from build123d import *

# Parameters (mm, degrees)
SKETCH_1_R          = 1.7
SKETCH_1_W          = 5
SKETCH_1_H          = 13
SKETCH_1_H_2        = 2
EXTRUDE_3_DEPTH     = 2.9
SKETCH_3_R          = 2.1
CUT_EXTRUDE_3_DEPTH = 2.9


with BuildPart() as part:
    # 草图1 → 凸台-拉伸3 (new body)
    # profile 1 of 10: a face of its own
    with BuildSketch(Plane(origin=(0, 0, 0), x_dir=(1, 0, 0), z_dir=(0, 1, 0))):
        with BuildLine():
            Line((-40, 113), (-70, 113))
            Line((-70, 113), (-70, 108))
            Line((-70, 108), (-70, 92))
            Line((-70, 92), (-63.7, 92))
            ThreePointArc((-63.7, 92), (-62, 93.7), (-60.3, 92))
            ThreePointArc((-60.3, 92), (-60.797918472, 90.797918472), (-62, 90.3))
            Line((-62, 90.3), (-62, 87))
            Line((-62, 87), (-48, 87))
            Line((-48, 87), (-48, 90.3))
            ThreePointArc((-48, 90.3), (-49.202081528, 93.202081528), (-46.3, 92))
            Line((-46.3, 92), (-40, 92))
            Line((-40, 92), (-40, 113))
        make_face()
        with Locations(Location((-62, 108, 0), (0, 0, 270))):
            Circle(SKETCH_1_R, mode=Mode.SUBTRACT)
        with Locations(Location((-48, 108, 0), (0, 0, 270))):
            Circle(SKETCH_1_R, mode=Mode.SUBTRACT)
    # profile 2 of 10: a face of its own
    with BuildSketch(Plane(origin=(0, 0, 0), x_dir=(1, 0, 0), z_dir=(0, 1, 0))):
        with BuildLine():
            Line((-70, 92), (-70, 87))
            Line((-70, 87), (-62, 87))
            Line((-62, 87), (-62, 90.3))
            ThreePointArc((-62, 90.3), (-63.202081528, 90.797918472), (-63.7, 92))
            Line((-63.7, 92), (-70, 92))
        make_face()
    # profile 3 of 10: a face of its own
    with BuildSketch(Plane(origin=(0, 0, 0), x_dir=(1, 0, 0), z_dir=(0, 1, 0))):
        with BuildLine():
            Line((-48, 90.3), (-48, 87))
            Line((-48, 87), (-40, 87))
            Line((-40, 87), (-40, 92))
            Line((-40, 92), (-46.3, 92))
            ThreePointArc((-46.3, 92), (-46.797918472, 90.797918472), (-48, 90.3))
        make_face()
    # profile 4 of 10: a face of its own
    with BuildSketch(Plane(origin=(0, 0, 0), x_dir=(1, 0, 0), z_dir=(0, 1, 0))):
        Polygon((-70, 87), (-70, 80), (-20, 80), (-20, 85), (-25, 85), (-25, 87), (-40, 87), (-48, 87), (-62, 87), align=None)
    # profile 5 of 10: a face of its own
    with BuildSketch(Plane(origin=(0, 0, 0), x_dir=(1, 0, 0), z_dir=(0, 1, 0))):
        Polygon((-25, 113), (-40, 113), (-40, 92), (-40, 87), (-25, 87), (-25, 100), align=None)
    # profile 6 of 10: a face of its own
    with BuildSketch(Plane(origin=(0, 0, 0), x_dir=(1, 0, 0), z_dir=(0, 1, 0))):
        with Locations((-22.5, 93.5)):
            Rectangle(SKETCH_1_W, SKETCH_1_H)
    # profile 7 of 10: a face of its own
    with BuildSketch(Plane(origin=(0, 0, 0), x_dir=(1, 0, 0), z_dir=(0, 1, 0))):
        with Locations((-22.5, 106.5)):
            Rectangle(SKETCH_1_W, SKETCH_1_H)
    # profile 8 of 10: a face of its own
    with BuildSketch(Plane(origin=(0, 0, 0), x_dir=(1, 0, 0), z_dir=(0, 1, 0))):
        with Locations((-22.5, 86)):
            Rectangle(SKETCH_1_W, SKETCH_1_H_2)
    # profile 9 of 10: a face of its own
    with BuildSketch(Plane(origin=(0, 0, 0), x_dir=(1, 0, 0), z_dir=(0, 1, 0))):
        Polygon((-20, 120), (-70, 120), (-70, 113), (-40, 113), (-25, 113), (-25, 115), (-20, 115), align=None)
    # profile 10 of 10: a face of its own
    with BuildSketch(Plane(origin=(0, 0, 0), x_dir=(1, 0, 0), z_dir=(0, 1, 0))):
        with Locations((-22.5, 114)):
            Rectangle(SKETCH_1_W, SKETCH_1_H_2)
    extrude(amount=EXTRUDE_3_DEPTH)

    # 草图3 → 切除-拉伸3 (cut)
    with BuildSketch(Plane(origin=(0, 2.9, 0), x_dir=(1, 0, 0), z_dir=(0, 1, 0))):
        with Locations(Location((-25, 110, 0), (0, 0, 270))):
            Circle(SKETCH_3_R)
        with Locations(Location((-25, 90, 0), (0, 0, 270))):
            Circle(SKETCH_3_R)
        with Locations(Location((-35, 90, 0), (0, 0, 270))):
            Circle(SKETCH_3_R)
        with Locations(Location((-35, 110, 0), (0, 0, 270))):
            Circle(SKETCH_3_R)
    extrude(amount=-CUT_EXTRUDE_3_DEPTH, mode=Mode.SUBTRACT)


solid = part.part
Verification items for the finished model (mm, model axes). Coordinates: 2 decimals unless noted, no trailing zeros. Order: outer loops, then holes, each group sorted by start corner. A loop starts at its lowest first (then second) coordinate and runs counter-clockwise, first axis right, second up. Notation, with made-up numbers: M 57.25,85 L 63.25,85 A23 cw 63.25,94 Z; hole C 18,-33.75 d5. An arc over 180 degrees is marked long. Return JSON: item names as keys, results as strings.
1) Gauge pin test, flat end, axial feed: pin 1 (2 mm diameter, centred on x = -48, z = -108, fed in from +Y). Record the tip position at first contact, or that the pin passes through.
Answer list:
{"pin 1": "through"}
2) Release check for a two-part mould opening along X. For faces 1 (the flat face through (-70, 1, -100)), 2 (the cylindrical face through (-23.23, 1.47, -108.87)), 3 (the flat face through (-45, 1, -80)) record: +X half, -X half, draft (parallel to the pull), parting line (faces both ways), or undercut.
Answer list:
{"face 1": "-X half", "face 2": "undercut", "face 3": "draft"}
3) Cross-section at A-A, the plane x = -35. Record the boundary of the cut face in (y, z).
Answer list:
{"outline": "M 0,-120 L 2.9,-120 L 2.9,-112.1 L 0,-112.1 Z; M 0,-107.9 L 2.9,-107.9 L 2.9,-92.1 L 0,-92.1 Z; M 0,-87.9 L 2.9,-87.9 L 2.9,-80 L 0,-80 Z"}
4) Cross-section at B-B, the plane y = 1.35. Count the separate pieces of the cut face and the enclosed holes in it, and give its area (3 significant figures).
Answer list:
{"separate pieces": "1", "enclosed holes": "8", "area": "1,910 mm2"}
5) Thickness scan on L1, parallel to X at y = 1.9, z = -110; L2, parallel to Z at x = -49, y = 0.9; L3, parallel to X at y = 2.3, z = -93. Record the ranges inside material, lowest first. Write a range as [from, to].
Answer list:
{"L1": "[-70, -37.1], [-32.9, -27.1], [-22.9, -20]", "L2": "[-120, -109.37], [-106.63, -93.37], [-90.63, -80]", "L3": "[-70, -63.37], [-60.63, -49.37], [-46.63, -20]"}
6) Cross-section at C-C, the plane z = -89.5. Record the boundary of the cut face in (x, y), and give its area (3 significant figures).
Answer list:
{"outline": "M -70,0 L -37.04,0 L -37.04,2.9 L -70,2.9 Z; M -32.96,0 L -27.04,0 L -27.04,2.9 L -32.96,2.9 Z; M -22.96,0 L -20,0 L -20,2.9 L -22.96,2.9 Z", "area": "121 mm2"}
